Geometry: final body of the model. Coordinates: model frame, mm. Round coordinates to 2 decimals unless told otherwise and drop trailing zeros. Write each loop counter-clockwise with the first axis right and the second up, starting at its lowest first coordinate (ties: lowest second). Pieces come first, ordered by that corner, then holes. Notation, with made-up numbers: M 7.25,-6.5 L 24.25,-6.5 A18 ccw 24.25,1.5 Z; hole C 43.25,-17 d10. An arc over 180 degrees is marked long. Put each result on its own line as item: value. Start each with the question number.
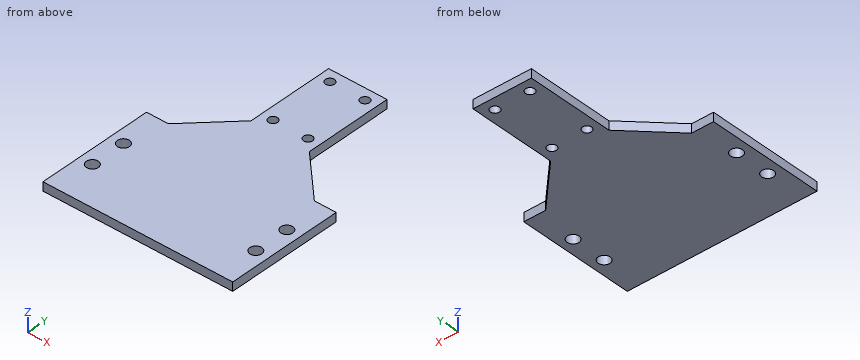
```python
from build123d import *

# Parameters (mm, degrees)
EXTRUDE_1_DEPTH     = 3
SKETCH_2_R          = 1.55
CUT_EXTRUDE_1_DEPTH = 92.050809991
SKETCH_3_R          = 2.05
CUT_EXTRUDE_2_DEPTH = 92.050809991


with BuildPart() as part:
    # 草图1 → 凸台-拉伸1 (new body)
    with BuildSketch(Plane.XY):
        Polygon((-32.5, 40), (-25, 40), (-10, 55), (-10, 85), (10, 85), (10, 55), (25, 40), (32.5, 40), (32.5, 0), (-32.5, 0), align=None)
    extrude(amount=EXTRUDE_1_DEPTH)

    # 草图2 → 切除-拉伸1 (cut, through all)
    with BuildSketch(Plane.XY.offset(3)):
        with Locations((-6, 81)):
            Circle(SKETCH_2_R)
        with Locations(Location((-6, 59, 0), (0, 0, 180))):
            Circle(SKETCH_2_R)
        with Locations((6, 59)):
            Circle(SKETCH_2_R)
        with Locations(Location((6, 81, 0), (0, 0, 180))):
            Circle(SKETCH_2_R)
    extrude(amount=-CUT_EXTRUDE_1_DEPTH, mode=Mode.SUBTRACT)

    # 草图3 → 切除-拉伸2 (cut, through all)
    with BuildSketch(Plane.XY.offset(3)):
        with Locations((-28, 26)):
            Circle(SKETCH_3_R)
        with Locations(Location((-28, 14, 0), (0, 0, 180))):
            Circle(SKETCH_3_R)
        with Locations((28, 14)):
            Circle(SKETCH_3_R)
        with Locations(Location((28, 26, 0), (0, 0, 180))):
            Circle(SKETCH_3_R)
    extrude(amount=-CUT_EXTRUDE_2_DEPTH, mode=Mode.SUBTRACT)


solid = part.part
```
1) Section C-C, the plane y = 81. Output: boundary loops of the cut face in (x, z), and give its area (3 significant figures).
2) First-contact query: pin 1 (3.5 mm diameter, centred on x = 6, y = 59, fed in from +Z); pin 2 (1.5 mm diameter, centred on y = 68, z = 1, fed in from +X); pin 3 (0.9 mm diameter, centred on x = -29.5, z = 1.5, fed in from +Y). Flat tips, straight axial feed; report the tip coordinate or a pass-through.
3) Section A-A, the plane x = 6. Output: boundary loops of the cut face in (y, z), and give its area (3 significant figures).
4) Section B-B, the plane z = 2.4. Give the number of separate pieces and of enclosed holes in the cut face, and give its area (3 significant figures).
5) Ray query, probe 1 along X at (y, z) = (81, 0.95); probe 2 along Y at (x, z) = (6, 1.85); probe 3 along Y at (x, z) = (28, 2.3). Return the intervals inside material, ascending.
6) Section D-D, the plane x = 17. Output: boundary loops of the cut face in (y, z).
Solved:
1. outline: M -10,0 L -7.55,0 L -7.55,3 L -10,3 Z; M -4.45,0 L 4.45,0 L 4.45,3 L -4.45,3 Z; M 7.55,0 L 10,0 L 10,3 L 7.55,3 Z
1. area: 41.4 mm2
2. pin 1: stops at z = 3
2. pin 2: stops at x = 10
2. pin 3: stops at y = 40
3. outline: M 0,0 L 57.45,0 L 57.45,3 L 0,3 Z; M 60.55,0 L 79.45,0 L 79.45,3 L 60.55,3 Z; M 82.55,0 L 85,0 L 85,3 L 82.55,3 Z
3. area: 236 mm2
4. separate pieces: 1
4. enclosed holes: 8
4. area: 3,640 mm2
5. probe 1: x = -10 to -7.55, -4.45 to 4.45, 7.55 to 10
5. probe 2: y = 0 to 57.45, 60.55 to 79.45, 82.55 to 85
5. probe 3: y = 0 to 11.95, 16.05 to 23.95, 28.05 to 40
6. outline: M 0,0 L 48,0 L 48,3 L 0,3 Z
